The model under review builds one solid part; all positions refer to its coordinate system, in mm. A direction names the side the tool comes from. Round coordinates to 2 decimals unless told otherwise and drop trailing zeros. Write each loop counter-clockwise with the first axis right and the second up, starting at its lowest first coordinate (ties: lowest second). Pieces come first, ordered by that corner, then holes. Notation, with made-up numbers: (-29, -36.5) - (-7, -36.5) arc R13 ccw to (-7, -31.5) - close; hole circle Ø10 at (-7, -35). An arc over 180 degrees is marked (long way). Use one line per item in the form item = value.
Autodesk Inventor part; units mm, degrees
ref_plane "FDT_CYLINDER_XY" through (0, 22, 0) normal (0, 1, 0) x (1, 0, 0)
ref_plane "FDT_CYLINDER_YZ" through (0, 22, 0) normal (1, 0, 0) x (0, 0, -1)
ref_plane "FDT_CYLINDER_ZX" through (0, 22, 0) normal (0, 0, -1) x (0, 1, 0)
sketch "Skizze_1" plane through (0, 0, 0) normal (0, 1, 0) x (-1, 0, 0)
  line L0 (25, 20) -> (-25, 20)
  line L1 (-25, 20) -> (-25, -20)
  line L2 (-25, -20) -> (25, -20)
  line L3 (25, -20) -> (25, 20)
  circle A0 centre (-20, -15) radius 2.75
  circle A1 centre (-20, 15) radius 2.75
  circle A2 centre (20, -15) radius 2.75
  circle A3 centre (20, 15) radius 2.75
extrude "Extrusion1" add sketch "Skizze_1" along normal blind 12
sketch "Skizze_2" plane through (0, 0, 0) normal (0, 0, 1) x (1, 0, 0)
  line L0 (0, -0.15) -> (0, 21.85)
  line L1 (0, 21.85) -> (8.5, 21.85)
  line L2 (8.5, 21.85) -> (8.5, 5.8)
  line L3 (8.5, 5.8) -> (13, 5.8)
  line L4 (13, 5.8) -> (13, -0.15)
  line L5 (13, -0.15) -> (0, -0.15)
  line L6 (0, -0.15) -> (0, 21.85)
revolve "Revolution1" add sketch "Skizze_2" angle 360 about axis through (0, -0.15, 0) along (0, -1, 0)
sketch "Skizze_3" plane through (0, 21.85, 0) normal (0, 1, 0) x (1, 0, 0)
  line L0 (-15, -15) -> (15, -15)
  line L1 (15, -15) -> (15, -7.5)
  line L2 (15, -7.5) -> (-13.5, -7.5)
  line L3 (-13.5, -7.5) -> (-13.5, 7.5)
  line L4 (-13.5, 7.5) -> (15, 7.5)
  line L5 (15, 7.5) -> (15, 15)
  line L6 (15, 15) -> (-15, 15)
  line L7 (-15, 15) -> (-15, -15)
extrude "Extrusion2" cut sketch "Skizze_3" along normal mid plane 17.6
sketch "Skizze_6" plane through (0, 0, 0) normal (0, 0, 1) x (1, 0, 0)
  line L0 (0, -0.15) -> (0, 21.85)
  line L1 (0, 21.85) -> (6, 21.85)
  line L2 (6, 21.85) -> (5.3235, 21.1735)
  line L3 (5.3235, 21.1735) -> (5.3235, 0.5265)
  line L4 (5.3235, 0.5265) -> (6, -0.15)
  line L5 (6, -0.15) -> (0, -0.15)
  line L6 (0, -0.15) -> (0, 21.85)
revolve "Revolution2" cut sketch "Skizze_6" angle 360 about axis through (0, -0.15, 0) along (0, -1, 0)
thread "Thread1"
ref_plane "FDT_CYLINDER_XY" through (0, 22, 0) normal (0, 1, 0) x (1, 0, 0)
ref_plane "FDT_CYLINDER_YZ" through (0, 22, 0) normal (1, 0, 0) x (0, 0, -1)
ref_plane "FDT_CYLINDER_ZX" through (0, 22, 0) normal (0, 0, -1) x (0, 1, 0)
properties part number "36126 KSZ-M12x1,25"
(1) To check wall thickness, follow L1, parallel to Z at x = -20, y = 7.5; L2, parallel to Y at x = -12.5, z = 11; L3, parallel to Y at x = 8.5, z = -9. State the ranges of each line that lie inside material, in increasing order.
Geometry results:
L1 = -20 to -17.75, -12.25 to 12.25, 17.75 to 20
L2 = 0 to 12
L3 = -0.15 to 12
(2) Add section C-C on x = 0. Write out the cut boundary in (y, z), then the cut area to 3 significant figures.
Geometry results:
outline = (-0.15, -13) - (0, -13) - (0, -20) - (12, -20) - (12, -8.5) - (13.05, -8.5) - (13.05, -7.5) - (21.85, -7.5) - (21.85, -6) - (21.17, -5.32) - (0.53, -5.32) - (-0.15, -6) - close; (-0.15, 6) - (0.53, 5.32) - (21.17, 5.32) - (21.85, 6) - (21.85, 7.5) - (13.05, 7.5) - (13.05, 8.5) - (12, 8.5) - (12, 20) - (0, 20) - (0, 13) - (-0.15, 13) - close
area = 399 mm2
(3) Machinability: for faces 1 (the flat face through (0, 12, 9)), 2 (the flat face through (0, 17, 7.5)), 3 (the flat face through (0, 17, -7.5)), which of the approach directions +Z, -Z, +X, -X, +Y, -Y give a long, thin tool a straight path to every point of the face, cutting with its end or side? Answer none if there is none.
Geometry results:
face_1 = +Y
face_2 = +Z, +X, -X, +Y
face_3 = -Z, +X, -X, +Y
(4) The part is to be moulded in two halves that separate along X. For faces 4 (the flat face through (-6, 21.85, 2)), 5 (the cylindrical face through (22.747, 5.916, -15.121)), 6 (the flat face through (-25, 6, 0)), say which applies: +X half, -X half, draft (parallel to the pull), parting line (faces both ways), or undercut.
Geometry results:
face_4 = draft
face_5 = undercut
face_6 = -X half
(5) Insertion check: P1, Ø5, axis at x = 9, y = 19, coming from the +Z side; P2, Ø2.5, axis at x = 1, y = 19.5, coming from the +Z side; P3, Ø12, axis at x = -0.5, y = 19.5, coming from the -Z side; P4, Ø5, axis at x = -20, z = -15, coming from the +Y side. Each pin has a flat end and moves straight along its axis. Give the tip position at first contact, or say it passes through.
Geometry results:
P1 = 5.48
P2 = 7.5
P3 = -7.5
P4 = through
(6) Add section A-A on z = -15. Write out the cut boundary in (x, y), then the cut area to 3 significant figures.
Geometry results:
outline = (-25, 0) - (-22.75, 0) - (-22.75, 12) - (-25, 12) - close; (-17.25, 0) - (17.25, 0) - (17.25, 12) - (-17.25, 12) - close; (22.75, 0) - (25, 0) - (25, 12) - (22.75, 12) - close
area = 468 mm2
(7) Add section B-B on y = 7.5. Write out the cut boundary in (x, z).
Geometry results:
outline = (-25, -20) - (25, -20) - (25, 20) - (-25, 20) - close; hole circle Ø5.5 at (-20, -15); hole circle Ø5.5 at (-20, 15); hole circle Ø10.65 at (0, 0); hole circle Ø5.5 at (20, -15); hole circle Ø5.5 at (20, 15)
(8) Add section D-D on z = 0. Write out the cut boundary in (x, y), then the cut area to 3 significant figures.
Geometry results:
outline = (-25, 0) - (-13, 0) - (-13, -0.15) - (-6, -0.15) - (-5.32, 0.53) - (-5.32, 21.17) - (-6, 21.85) - (-8.5, 21.85) - (-8.5, 12) - (-25, 12) - close; (5.32, 0.53) - (6, -0.15) - (13, -0.15) - (13, 0) - (25, 0) - (25, 12) - (8.5, 12) - (8.5, 21.85) - (6, 21.85) - (5.32, 21.17) - close
area = 536 mm2
